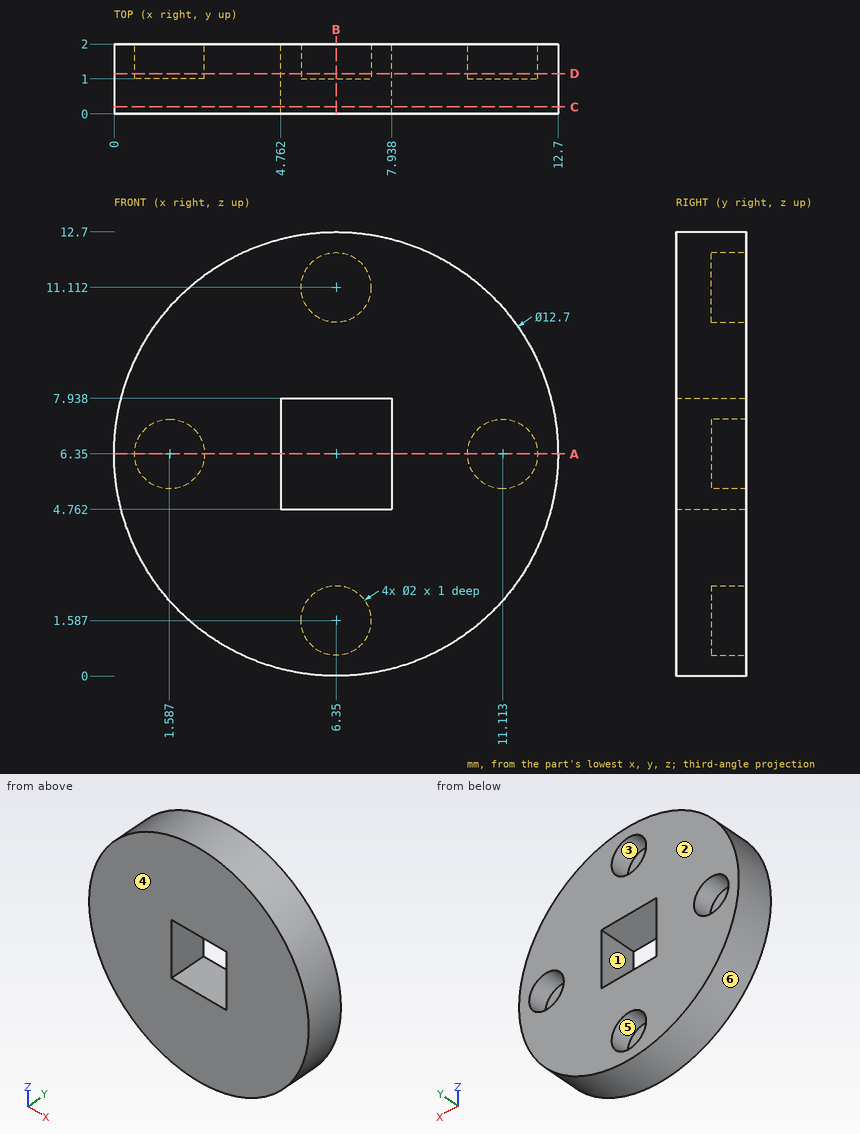
Design review of the part shown in the three views and the two pictorial views. Dimensions are in mm from the part's minimum x, y and z. A direction names the side the tool comes from. Round coordinates to 2 decimals unless told otherwise and drop trailing zeros. Loops run counter-clockwise (first coordinate to the right, second up) from the corner with the lowest first, then second, coordinate; pieces in that order, holes last. Notation, with made-up numbers: (-39, 35.5) - (-2, 35.5) arc R18 cw to (-2, 64.5) - close; hole circle Ø8 at (-7.75, 80). An arc over 180 degrees is marked (long way). Write each question's results on one line, items separated by ' | '. Start each with the question number.
Q1. Draft analysis for pull direction X (two halves, no side actions). For the marked faces 4, 5 and 6, state which applies: pulls with the +X half, pulls with the -X half, needs draft (parallel to the pull), parting line crosses it, or undercut.
Q2. Take a section at B-B on x = 6.35. Give the boundary of the cut face in (y, z).
Q3. Take a section at D-D on y = 1.15. Give the boundary of the cut face in (x, z).
Q4. Take a section at C-C on y = 0.2. Give the boundary of the cut face in (x, z), plus the area to 3 significant figures.
Q5. Insertion check: P1, Ø1, axis at x = 11, z = 6.5, coming from the +Y side; P2, Ø0.6, axis at y = 1, z = 7, coming from the -X side. Each pin has a flat end and moves straight along its axis. Give the tip position at first contact, or say it passes through.
Q6. Tool access review of the marked faces 1, 2 and 3: name each direction out of +Z, -Z, +X, -X, +Y, -Y from which nothing blocks a thin tool from reaching the whole face with its end or side.
Q7. Take a section at A-A on z = 6.35. Give the boundary of the cut face in (x, y).
Q8. Wall thickness on line 1 along X through (y, z) = (1.4, 6.35); line 2 along Z through (x, y) = (6.5, 1.05) (1 decimal); line 3 along X through (y, z) = (0.5, 5.75): over which ranges is each line inside the solid? List them lowest first. Write a range as [from, to].
Data:
1) face 4: needs draft | face 5: undercut | face 6: parting line crosses it
2) outline: (0, 0) - (2, 0) - (2, 0.59) - (1, 0.59) - (1, 2.59) - (2, 2.59) - (2, 4.76) - (0, 4.76) - close; (0, 7.94) - (2, 7.94) - (2, 10.11) - (1, 10.11) - (1, 12.11) - (2, 12.11) - (2, 12.7) - (0, 12.7) - close
3) outline: circle Ø12.7 at (6.35, 6.35); hole circle Ø2 at (1.59, 6.35); hole (4.76, 4.76) - (7.94, 4.76) - (7.94, 7.94) - (4.76, 7.94) - close; hole circle Ø2 at (6.35, 1.59); hole circle Ø2 at (6.35, 11.11); hole circle Ø2 at (11.11, 6.35)
4) outline: circle Ø12.7 at (6.35, 6.35); hole (4.76, 4.76) - (7.94, 4.76) - (7.94, 7.94) - (4.76, 7.94) - close | area: 117 mm²
5) P1: stops at y = 1 | P2: stops at x = 0.01
6) face 1: +Y, -Y | face 2: +Z, -Z, +X, -X, +Y | face 3: +Y
7) outline: (0, 0) - (4.76, 0) - (4.76, 2) - (2.59, 2) - (2.59, 1) - (0.59, 1) - (0.59, 2) - (0, 2) - close; (7.94, 0) - (12.7, 0) - (12.7, 2) - (12.11, 2) - (12.11, 1) - (10.11, 1) - (10.11, 2) - (7.94, 2) - close
8) line 1: x = [0, 0.59], [2.59, 4.76], [7.94, 10.11], [12.11, 12.7] | line 2: z = [0, 0.6], [2.6, 4.8], [7.9, 10.1], [12.1, 12.7] | line 3: x = [0.03, 4.76], [7.94, 12.67]
